Source: CAD feature listing. Evaluate the final solid. Frame: model axes, mm. A direction names the side the tool comes from. Round coordinates to 2 decimals unless told otherwise and drop trailing zeros. Loops run counter-clockwise (first coordinate to the right, second up) from the corner with the lowest first, then second, coordinate; pieces in that order, holes last.
Item 1: Ray query, L1, parallel to Y at x = -0.1, z = 0 (3 decimals); L2, parallel to Y at x = -0.6, z = -0.75; L3, parallel to X at y = -2.5, z = 1.1. Return the intervals inside material, ascending.
Item 2: Access query for faces 1 (the flat face through (0.25, -1, 0)), 2 (the flat face through (0, 1, -2)), 3 (the flat face through (-0.5, 1, 0)). Directions: +Z, -Z, +X, -X, +Y, -Y. A direction counts if a zero-diameter tool reaches every point of the face in a straight line with its end or side. Return the directions, or none.
Item 3: Pull-direction query (Y, two-part tool) for faces 4 (the flat face through (0, 3, 0)), 5 (the flat face through (-0.25, -1, 0)), 6 (the cylindrical face through (0, -1.41, 0.13)); classes: released by +Y, released by -Y, zero draft, split by the parting line, or undercut.
Item 4: Section query B-B on y = 1.5. Return loops of the section in (x, z) (3 decimals).
Item 5: Section query A-A on x = 0. Return loops of the section in (y, z) (3 decimals).
Item 6: Section query C-C on z = 0. Give the number of separate pieces and of enclosed holes in the cut face, then the cut area to 3 significant figures.
Item 7: First-contact query: P1, Ø0.9, axis at y = -1.5, z = 0.5, coming from the -X side; P2, Ø0.6, axis at y = 1.5, z = 1, coming from the -X side; P3, Ø0.6, axis at x = 0, y = -1.5, coming from the -Z side. Flat tips, straight axial feed; report the tip coordinate or a pass-through.
```python
from build123d import *

# Parameters (mm, degrees)
SZKIC1_W                    = 1
SZKIC1_H                    = 4
DODANIE_WYCI_GNI_CIE1_DEPTH = 3
SZKIC4_W                    = 0.5
SZKIC4_H                    = 3
DODANIE_WYCI_GNI_CIE3_DEPTH = 3.9
SZKIC5_R                    = 1
WYTNIJ_WYCI_GNI_CIE2_DEPTH  = 3.9
ZAOKR_GLENIE1_R             = 0.25
SZKIC8_W                    = 4
SZKIC8_H                    = 1
DODANIE_WYCI_GNI_CIE4_DEPTH = 0.5
SZKIC9_R                    = 0.125
WYTNIJ_WYCI_GNI_CIE3_DEPTH  = 1


with BuildPart() as part:
    # Szkic1 → Dodanie-wyciągnięcie1 (new body)
    with BuildSketch(Plane(origin=(0, 0, 0), x_dir=(1, 0, 0), z_dir=(0, 1, 0))):
        Rectangle(SZKIC1_W, SZKIC1_H)
    extrude(amount=DODANIE_WYCI_GNI_CIE1_DEPTH)

    # Szkic4 → Dodanie-wyciągnięcie3 (add)
    with BuildSketch(Plane.XZ):
        Rectangle(SZKIC4_W, SZKIC4_H)
    extrude(amount=DODANIE_WYCI_GNI_CIE3_DEPTH)

    # Szkic5 → Wytnij-wyciągnięcie2 (cut)
    with BuildSketch(Plane(origin=(0.25, 0, 0), x_dir=(0, 0, -1), z_dir=(1, 0, 0))):
        with Locations((0, -2.4)):
            Circle(SZKIC5_R)
    extrude(amount=-WYTNIJ_WYCI_GNI_CIE2_DEPTH, mode=Mode.SUBTRACT)

    # Zaokrąglenie1
    zaokr_glenie1_edges = [part.edges().sort_by_distance(p)[0] for p in [
        (0.25, 0, 0),
        (0, 0, 1.5),
        (-0.25, 0, 0),
        (0, 0, -1.5),
        (0, -3.9, 1.5),
        (0, -3.9, -1.5),
    ]]
    fillet(zaokr_glenie1_edges, radius=ZAOKR_GLENIE1_R - 0.0001)  # a hair under: the kernel refuses the full size

    # Szkic8 → Dodanie-wyciągnięcie4 (add)
    with BuildSketch(Plane.ZY.offset(0.5)):
        with Locations((0, 2.5)):
            Rectangle(SZKIC8_W, SZKIC8_H)
    extrude(amount=DODANIE_WYCI_GNI_CIE4_DEPTH)

    # Szkic9 → Wytnij-wyciągnięcie3 (cut)
    with BuildSketch(Plane(origin=(0.5, 0, 0), x_dir=(0, 0, -1), z_dir=(1, 0, 0))):
        with Locations((0, 1.5)):
            Circle(SZKIC9_R)
    extrude(amount=-WYTNIJ_WYCI_GNI_CIE3_DEPTH, mode=Mode.SUBTRACT)


solid = part.part
```
Data:
1. L1: y = -3.9 to -3.4, -1.4 to 1.375, 1.625 to 3
1. L2: y = 2 to 3
1. L3: x = -0.25 to 0.25
2. face 1: +Z, -Z, +X, -Y
2. face 2: -Z, +X, -X, +Y, -Y
2. face 3: +Z, -Z, -X, -Y
3. face 4: released by +Y
3. face 5: zero draft
3. face 6: undercut
4. outline: (-0.5, -2) - (0.5, -2) - (0.5, -0.125) - (-0.5, -0.125) - close; (-0.5, 0.125) - (0.5, 0.125) - (0.5, 2) - (-0.5, 2) - close
5. outline: (-3.9, -1.25) arc R0.25 ccw to (-3.65, -1.5) - (-0.25, -1.5) arc R0.25 cw to (0, -1.75) - (0, -2) - (3, -2) - (3, 2) - (0, 2) - (0, 1.75) arc R0.25 cw to (-0.25, 1.5) - (-3.65, 1.5) arc R0.25 ccw to (-3.9, 1.25) - close; hole circle Ø2 at (-2.4, 0); hole circle Ø0.25 at (1.5, 0)
6. separate pieces: 3
6. enclosed holes: 0
6. area: 4.23 mm2
7. P1: stops at x = -0.25
7. P2: stops at x = -0.5
7. P3: stops at z = -1.5
